Autodesk Inventor part; units mm, degrees
ref_plane "YZ Plane" through (0, 0, 0) normal (1, 0, 0) x (0, 1, 0)
ref_plane "XZ Plane" through (0, 0, 0) normal (0, 1, 0) x (-1, 0, 0)
ref_plane "XY Plane" through (0, 0, 0) normal (0, 0, 1) x (1, 0, 0)
sketch "Boceto1" plane through (0, 0, 0) normal (0, 1, 0) x (-1, 0, 0)
  line L0 (-10, 10) -> (10, 10)
  line L1 (10, 10) -> (10, -10)
  line L2 (10, -10) -> (-10, -10)
  line L3 (-10, -10) -> (-10, 10)
  line L4 (-10, 10) -> (10, -10) construction
  line L5 (10, 10) -> (-10, -10) construction
  line L6 (10, 22) -> (-10, 22)
  line L7 (-10, 22) -> (-10, -22)
  line L8 (-10, -22) -> (10, -22)
  line L9 (10, -22) -> (10, 22)
  circle A0 centre (0, 16) radius 2.7
  circle A1 centre (0, -16) radius 2.7
  point P0 (0, 0)
  dimension "d0" = 20
  dimension "d1" = 20
  dimension "d2" = 5.4
  dimension "d3" = 5.4
  dimension "d4" = 6
  dimension "d5" = 6
  dimension "d6" = 6
  dimension "d7" = 6
extrude "Extrusión1" add sketch "Boceto1" along normal blind 17
sketch "Boceto2" plane through (0, 17, 0) normal (0, 1, 0) x (1, 0, 0)
  circle A0 centre (-3, -4.75) radius 1.2
  circle A1 centre (-3, 4.75) radius 1.2
  line L0 (-10, 22) -> (-10, -22)
  point P0 (0, 0)
  dimension "d10" = 2.4
  dimension "d11" = 9.5
  dimension "d12" = 4.75
  dimension "d13" = 7
extrude "Extrusión2" cut sketch "Boceto2" against normal through all
sketch "Boceto3" plane through (0, 17, 0) normal (0, 1, 0) x (1, 0, 0)
  line L0 (-10, 22) -> (-10, -22)
  line L1 (10, -10) -> (-10, -10)
  line L2 (-10, -10) -> (-10, 10)
  line L3 (-10, 10) -> (10, 10)
  line L4 (10, 10) -> (10, -10)
  line L5 (10, -10) -> (-10, 10) construction
  line L6 (-10, -10) -> (10, 10) construction
  circle A0 centre (-3, 4.75) radius 1.2
  circle A1 centre (-3, -4.75) radius 1.2
  line L7 (10, -22) -> (10, 22)
  line L8 (10, 22) -> (-10, 22)
  line L9 (-10, 22) -> (-10, -22)
  line L10 (-10, -22) -> (10, -22)
  circle A2 centre (0, -16) radius 2.7
  circle A3 centre (0, 16) radius 2.7
  point P0 (0, 0)
  point P1 (-10, -22)
  point P2 (-10, -10)
  dimension "d16" = 20
extrude "Extrusión3" cut sketch "Boceto3" against normal blind 13 contours L8 L7 L3 L0 | L1 L7 L10 L0
sketch "Boceto4" plane through (0, 4, 0) normal (0, 1, 0) x (1, 0, 0)
  circle A0 centre (0, -16) radius 2.7
  circle A1 centre (0, -16) radius 4.7
  circle A2 centre (0, 16) radius 2.7
  circle A3 centre (0, 16) radius 4.7
  point P0 (0, 0)
  dimension "d19" = 9.4
extrude "Extrusión4" cut sketch "Boceto4" against normal blind 1
sketch "Boceto5" plane through (0, 17, 0) normal (0, 1, 0) x (1, 0, 0)
  line L0 (-10, -10) -> (10, -10)
  line L1 (10, 10) -> (-10, 10)
  line L2 (10, -10) -> (0, -10)
  line L3 (0, -10) -> (0, 10)
  line L4 (0, 10) -> (10, 10)
  line L5 (10, 10) -> (10, -10)
  point P0 (0, 0)
  point P1 (0, -10)
  dimension "d22" = 10
extrude "Extrusión5" cut sketch "Boceto5" against normal up to surface (13 mm away)
fillet "Empalme1" radius 2 4 edges at (10, 2, 22) (-10, 2, 22) (10, 2, -22) (-10, 2, -22)
fillet "Empalme2" radius 5 1 edges at (0, 4, 0)
fillet "Empalme3" radius 2 6 edges at (-10, 10.5, 10) (-10, 10.5, -10) (0, 13, 10) (0, 13, -10) (1.4645, 5.4645, -10) (1.4645, 5.4645, 10)
sketch "Boceto6" plane through (0, 0, 0) normal (0, -1, 0) x (1, 0, 0)
  circle A0 centre (-3, -4.75) radius 1.2
  circle A1 centre (-3, -4.75) radius 2.15
  circle A2 centre (-3, 4.75) radius 1.2
  circle A3 centre (-3, 4.75) radius 2.15
  line L0 (-5.4826, -4.75) -> (-4.2413, -2.6)
  line L1 (-4.2413, -2.6) -> (-1.7587, -2.6)
  line L2 (-1.7587, -2.6) -> (-0.5174, -4.75)
  line L3 (-0.5174, -4.75) -> (-1.7587, -6.9)
  line L4 (-1.7587, -6.9) -> (-4.2413, -6.9)
  line L5 (-4.2413, -6.9) -> (-5.4826, -4.75)
  line L6 (-5.4826, 4.75) -> (-4.2413, 6.9)
  line L7 (-4.2413, 6.9) -> (-1.7587, 6.9)
  line L8 (-1.7587, 6.9) -> (-0.5174, 4.75)
  line L9 (-0.5174, 4.75) -> (-1.7587, 2.6)
  line L10 (-1.7587, 2.6) -> (-4.2413, 2.6)
  line L11 (-4.2413, 2.6) -> (-5.4826, 4.75)
  point P0 (0, 0)
  dimension "d29" = 4.3
  dimension "d30" = 4.3
extrude "Extrusión6" cut sketch "Boceto6" against normal blind 15 contours A0 | A1 | A1 L2 L3 | A1 L1 L2 | L3 L4 A1 | A1 L0 L1 | L4 L5 A1 | A1 L5 L0 | A2 | A3 | A3 L8 L9 | A3 L7 L8 | L9 L10 A3 | A3 L6 L7 | L10 L11 A3 | A3 L11 L6
properties part number "soporteendstop"
Can you work these out from the model? Positions are in its coordinate system, mm. A direction names the side the tool comes from. Round coordinates to 2 decimals unless told otherwise and drop trailing zeros. Loops run counter-clockwise (first coordinate to the right, second up) from the corner with the lowest first, then second, coordinate; pieces in that order, holes last. Notation, with made-up numbers: (21.5, 65.25) -> (49.5, 65.25) arc R19 cw to (49.5, 101.25) -> close; hole circle Ø3 at (-23.75, 82.5). An arc over 180 degrees is marked (long way). One line per item, written item: value. Start each with the question number.
1. If we section it at A-A, the plane z = 16: Write out the boundary of the cut face in (x, y).
2. If I drill on probe 1 along Z at (x, y) = (-3, 15.4); probe 2 along X at (y, z) = (3.75, -16); probe 3 along Z at (x, y) = (-3.25, 13.25), over which ranges is the centre line in solid material (lowest first)?
3. If we section it at C-C, the plane z = 0.5: Write out the boundary of the cut face in (x, y), then the cut area to 3 significant figures.
4. If we mould it in two halves opening along Z, with no side actions, what happens to faces 1 (the flat face through (-5, 11, -10)), 2 (the flat face through (-4.87, 7.4, 5.81)), 3 (the cylindrical face through (-4.2, 16, 4.7)), 4 (the flat face through (-5, 11, 10))? For each: pulls with the +Z half, pulls with the -Z half, needs draft (parallel to the pull), parting line crosses it, or undercut.
5. For faces 5 (the flat face through (0, 13, 0)), 6 (the flat face through (-3, 7, -6.9)), 7 (the cylindrical face through (-0.57, 12.94, 9.4)), 8 (the cylindrical face through (-0.57, 13.06, -9.4)), 9 (the cylindrical face through (-1.02, 3.51, 20.59)), which set-ups out of +Z, -Z, +X, -X, +Y, -Y let a thin tool reach every point of the face, with its end or its side?
6. For pin 1 (11 mm diameter, centred on x = 0, z = -16, fed in from +Y); pin 2 (2 mm diameter, centred on x = -2.5, z = -5.5, fed in from -Y); pin 3 (2 mm diameter, centred on x = -2.5, y = 9.5, fed in from -Z), each with a flat end and sliding along its axis, tell me the tip position at first contact or that it passes through.
7. If we section it at B-B, the plane x = -6.25: Write out the boundary of the cut face in (y, z), then the cut area to 3 significant figures.
8. If we section it at D-D, the plane y = 5: Give the number of separate pieces and of enclosed holes in the cut face, then the cut area to 3 significant figures.
Calculated:
1. outline: (-10, 0) -> (-2.7, 0) -> (-2.7, 3) -> (-4.7, 3) -> (-4.7, 4) -> (-10, 4) -> close; (2.7, 0) -> (10, 0) -> (10, 4) -> (4.7, 4) -> (4.7, 3) -> (2.7, 3) -> close
2. probe 1: z = -10 to -5.95, -3.55 to 3.55, 5.95 to 10
2. probe 2: x = -10 to -4.7, 4.7 to 10
2. probe 3: z = -10 to -6.9, -2.6 to 2.6, 6.9 to 10
3. outline: (-10, 0) -> (10, 0) -> (10, 4) -> (5, 4) arc R5 cw to (0, 9) -> (0, 17) -> (-10, 17) -> close
3. area: 215 mm²
4. face 1: pulls with the -Z half
4. face 2: undercut
4. face 3: undercut
4. face 4: pulls with the +Z half
5. face 5: +Z, -Z, +X, +Y
5. face 6: -Y
5. face 7: +Z, +X, +Y
5. face 8: -Z, +X, +Y
5. face 9: +Y
6. pin 1: stops at y = 4
6. pin 2: stops at y = 15
6. pin 3: stops at z = -10
7. outline: (0, -22) -> (4, -22) -> (4, -10) -> (17, -10) -> (17, 10) -> (4, 10) -> (4, 22) -> (0, 22) -> close
7. area: 436 mm²
8. separate pieces: 1
8. enclosed holes: 2
8. area: 204 mm²
